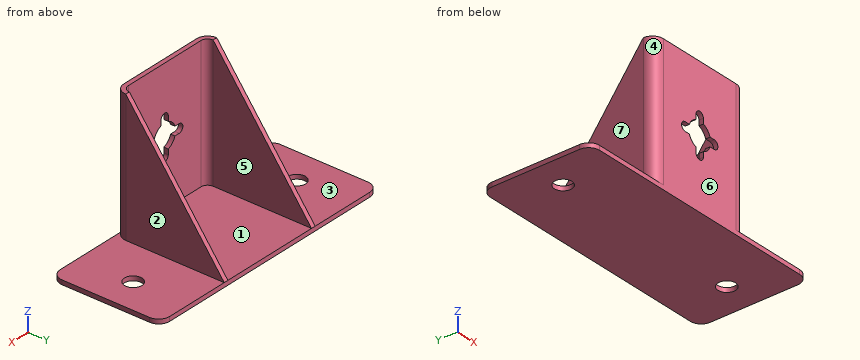
```python
from build123d import *

# Parameters (mm, degrees)
SALIENTE_EXTRUIR1_DEPTH = 2
SALIENTE_EXTRUIR2_DEPTH = 60
CORTAR_EXTRUIR1_DEPTH   = 50
CROQUIS4_R              = 4
CORTAR_EXTRUIR2_DEPTH   = 2
CORTAR_EXTRUIR6_DEPTH   = 2


with BuildPart() as part:
    # Croquis1 → Saliente-Extruir1 (new body)
    with BuildSketch(Plane.XY):
        with BuildLine():
            Line((-55, -25), (55, -25))
            ThreePointArc((55, -25), (58.535533906, -23.535533906), (60, -20))
            Line((60, -20), (60, 20))
            ThreePointArc((60, 20), (58.535533906, 23.535533906), (55, 25))
            Line((55, 25), (-55, 25))
            ThreePointArc((-55, 25), (-58.535533906, 23.535533906), (-60, 20))
            Line((-60, 20), (-60, -20))
            ThreePointArc((-60, -20), (-58.535533906, -23.535533906), (-55, -25))
        make_face()
    extrude(amount=SALIENTE_EXTRUIR1_DEPTH)

    # Croquis2 → Saliente-Extruir2 (add)
    with BuildSketch(Plane.XY.offset(2)):
        with BuildLine():
            Line((-20, -25), (20, -25))
            ThreePointArc((20, -25), (23.535533906, -23.535533906), (25, -20))
            Line((25, -20), (25, 25))
            Line((25, 25), (23, 25))
            Line((23, 25), (23, -20))
            ThreePointArc((23, -20), (22.121320344, -22.121320344), (20, -23))
            Line((20, -23), (-20, -23))
            ThreePointArc((-20, -23), (-22.121320344, -22.121320344), (-23, -20))
            Line((-23, -20), (-23, 25))
            Line((-23, 25), (-25, 25))
            Line((-25, 25), (-25, -20))
            ThreePointArc((-25, -20), (-23.535533906, -23.535533906), (-20, -25))
        make_face()
    extrude(amount=SALIENTE_EXTRUIR2_DEPTH)

    # Croquis3 → Cortar-Extruir1 (cut)
    with BuildSketch(Plane(origin=(25, 0, 0), x_dir=(0, 0, -1), z_dir=(1, 0, 0))):
        Polygon((-62, -20), (-2, 25), (-62, 25), align=None)
    extrude(amount=-CORTAR_EXTRUIR1_DEPTH, mode=Mode.SUBTRACT)

    # Croquis4 → Cortar-Extruir2 (cut)
    with BuildSketch(Plane(origin=(0, 0, 0), x_dir=(-1, 0, 0), z_dir=(0, 0, -1))):
        with Locations((-45, 0)):
            Circle(CROQUIS4_R)
        with Locations((45, 0)):
            Circle(CROQUIS4_R)
    extrude(amount=-CORTAR_EXTRUIR2_DEPTH, mode=Mode.SUBTRACT)

    # Croquis5 → Cortar-Extruir6 (cut)
    with BuildSketch(Plane.XZ.offset(25)):
        with BuildLine():
            ThreePointArc((-2, 23.499997), (0, 21.499997), (2, 23.499997))
            Line((2, 23.499997), (2, 25.84314275))
            ThreePointArc((2, 25.84314275), (4.242640687, 27.257356313), (5.656854249, 29.499997))
            Line((5.656854249, 29.499997), (8, 29.499997))
            ThreePointArc((8, 29.499997), (10, 31.499997), (8, 33.499997))
            Line((8, 33.499997), (5.656854249, 33.499997))
            ThreePointArc((5.656854249, 33.499997), (4.242640687, 35.742637687), (2, 37.156851249))
            Line((2, 37.156851249), (2, 39.499997))
            ThreePointArc((2, 39.499997), (0, 41.499997), (-2, 39.499997))
            Line((-2, 39.499997), (-2, 37.156851249))
            ThreePointArc((-2, 37.156851249), (-4.242640687, 35.742637687), (-5.656854249, 33.499997))
            Line((-5.656854249, 33.499997), (-8, 33.499997))
            ThreePointArc((-8, 33.499997), (-10, 31.499997), (-8, 29.499997))
            Line((-8, 29.499997), (-5.656854249, 29.499997))
            ThreePointArc((-5.656854249, 29.499997), (-4.242640687, 27.257356313), (-2, 25.84314275))
            Line((-2, 25.84314275), (-2, 23.499997))
        make_face()
    extrude(amount=-CORTAR_EXTRUIR6_DEPTH, mode=Mode.SUBTRACT)


solid = part.part
```
Can you work these out from the model? Positions are in its coordinate system, mm. Face numbers are marked on the shaded views. A direction names the side the tool comes from. Round coordinates to 2 decimals unless told otherwise and drop trailing zeros. Loops run counter-clockwise (first coordinate to the right, second up) from the corner with the lowest first, then second, coordinate; pieces in that order, holes last. Notation, with made-up numbers: (55.5, 81.5) -> (61.5, 81.5) arc R23 cw to (61.5, 119.5) -> close; hole circle Ø3 at (4, -12). An arc over 180 degrees is marked (long way). Answer in a Markdown table with one row per item.
Item 1: On a 3-axis mill with a long thin cutter (end or side, diameter ignored), from which of +Z, -Z, +X, -X, +Y, -Y can I reach the whole of each face in a straight line? I mean the marked faces 5, 6 and 7. Say none if no direction works.
Answer block:
| item | result |
|---|---|
| face 5 | +Z, +Y |
| face 6 | +Z, -Z, +X, -X, -Y |
| face 7 | +Z, -X, +Y, -Y |
Item 2: Suppose I cut it at D-D, the plane x = 0. List the corners of the cut face in (y, z) for me, plus the area to 3 significant figures.
Answer block:
| item | result |
|---|---|
| outline | (-25, 0) -> (25, 0) -> (25, 2) -> (-23, 2) -> (-23, 21.5) -> (-25, 21.5) -> close; (-25, 41.5) -> (-23, 41.5) -> (-23, 62) -> (-25, 62) -> close |
| area | 180 mm² |
Item 3: Will these pins go through, and if not, where does the flat tip stop? P1, Ø13.5, axis at y = 6.5, z = 28.5, coming from the -X side; P2, Ø4, axis at y = -19.5, z = 19.5, coming from the +X side; P3, Ø8, axis at x = -18.5, z = 31, coming from the +Y side.
Answer block:
| item | result |
|---|---|
| P1 | x = -25 |
| P2 | x = 25 |
| P3 | y = -21.66 |
Item 4: Suppose I cut it at C-C, the plane y = 7. List the corners of the cut face in (x, z) for me, plus the area to 3 significant figures.
Answer block:
| item | result |
|---|---|
| outline | (-60, 0) -> (60, 0) -> (60, 2) -> (25, 2) -> (25, 26) -> (23, 26) -> (23, 2) -> (-23, 2) -> (-23, 26) -> (-25, 26) -> (-25, 2) -> (-60, 2) -> close |
| area | 336 mm² |
Item 5: If I drill on probe 1 along X at (y, z) = (0.5, 18); probe 2 along Y at (x, z) = (-45, 1); probe 3 along Z at (x, y) = (22, 20), over which ranges is the centre line in solid material (lowest first)?
Answer block:
| item | result |
|---|---|
| probe 1 | -25 to -23, 23 to 25 |
| probe 2 | -25 to -4, 4 to 25 |
| probe 3 | 0 to 2 |
Item 6: We'd pull the mould along X, two halves only. Please class the marked faces 1, 2, 3 and 4: released by +X, released by -X, zero draft, split by the parting line, or undercut.
Answer block:
| item | result |
|---|---|
| face 1 | undercut |
| face 2 | released by +X |
| face 3 | zero draft |
| face 4 | released by -X |
Item 7: Suppose I cut it at B-B, the plane z = 50. List the corners of the cut face in (x, y) for me, plus the area to 3 significant figures.
Answer block:
| item | result |
|---|---|
| outline | (-25, -20) arc R5 ccw to (-20, -25) -> (20, -25) arc R5 ccw to (25, -20) -> (25, -11) -> (23, -11) -> (23, -20) arc R3 cw to (20, -23) -> (-20, -23) arc R3 cw to (-23, -20) -> (-23, -11) -> (-25, -11) -> close |
| area | 141 mm² |
Item 8: Suppose I cut it at A-A, the plane x = 45. List the corners of the cut face in (y, z) for me.
Answer block:
| item | result |
|---|---|
| outline | (-25, 0) -> (-4, 0) -> (-4, 2) -> (-25, 2) -> close; (4, 0) -> (25, 0) -> (25, 2) -> (4, 2) -> close |
